Source: CAD feature listing. Evaluate the final solid. Frame: model axes, mm. A direction names the side the tool comes from. Give positions to 0.01 mm unless a question says otherwise; leave off trailing zeros. Loops run counter-clockwise (first coordinate to the right, second up) from the corner with the lowest first, then second, coordinate; pieces in that order, holes last.
from build123d import *

# Parameters (mm, degrees)
SKETCH_1_W          = 110
SKETCH_1_H          = 110
EXTRUDE_1_DEPTH     = 9
SKETCH_2_R          = 6.2
CUT_EXTRUDE_1_DEPTH = 9
SKETCH_10_W         = 8
SKETCH_10_H         = 8
CUT_EXTRUDE_3_DEPTH = 10
SKETCH_9_W          = 110
SKETCH_9_H          = 15
CUT_EXTRUDE_4_DEPTH = 10
FILLET_1_R          = 10
SKETCH_11_W         = 8
SKETCH_11_H         = 3
CUT_EXTRUDE_5_DEPTH = 10
SKETCH_12_R         = 1.7
CUT_EXTRUDE_6_DEPTH = 10


with BuildPart() as part:
    # 草图1 → 凸台-拉伸1 (new body)
    with BuildSketch(Plane(origin=(0, 0, 0), x_dir=(1, 0, 0), z_dir=(0, 1, 0))):
        with BuildLine():
            Line((-98.584118364, 105), (98.584118364, 105))
            ThreePointArc((98.584118364, 105), (103.984134744, 103.416639656), (107.674116766, 99.167964619))
            Line((107.674116766, 99.167964619), (147.029996803, 13.335929237))
            ThreePointArc((147.029996803, 13.335929237), (148.644315385, 2.139042389), (143.925625878, -8.142507538))
            Line((143.925625878, -8.142507538), (92.989084735, -66.571253769))
            ThreePointArc((92.989084735, -66.571253769), (89.591770698, -69.102541889), (85.451271796, -70))
            Line((85.451271796, -70), (50, -70))
            Line((50, -70), (-55, -70))
            Line((-55, -70), (-85.451271796, -70))
            ThreePointArc((-85.451271796, -70), (-89.591770698, -69.102541889), (-92.989084735, -66.571253769))
            Line((-92.989084735, -66.571253769), (-143.925625878, -8.142507538))
            ThreePointArc((-143.925625878, -8.142507538), (-148.644315385, 2.139042389), (-147.029996803, 13.335929237))
            Line((-147.029996803, 13.335929237), (-107.674116766, 99.167964619))
            ThreePointArc((-107.674116766, 99.167964619), (-103.984134744, 103.416639656), (-98.584118364, 105))
        make_face()
        Rectangle(SKETCH_1_W, SKETCH_1_H, mode=Mode.SUBTRACT)
    extrude(amount=EXTRUDE_1_DEPTH)

    # 草图2 → 切除-拉伸1 (cut)
    with BuildSketch(Plane(origin=(0, 9, 0), x_dir=(1, 0, 0), z_dir=(0, 1, 0))):
        with Locations(Location((-128.85, 5, 0), (0, 0, 270))):
            Circle(SKETCH_2_R)
        with Locations(Location((128.85, 5, 0), (0, 0, 270))):
            Circle(SKETCH_2_R)
    extrude(amount=-CUT_EXTRUDE_1_DEPTH, mode=Mode.SUBTRACT)

    # 草图10 → 切除-拉伸3 (cut)
    with BuildSketch(Plane(origin=(0, 9, 0), x_dir=(1, 0, 0), z_dir=(0, 1, 0))):
        with Locations((-59, 0)):
            Rectangle(SKETCH_10_W, SKETCH_10_H)
        with Locations((0, 59)):
            Rectangle(SKETCH_10_W, SKETCH_10_H)
        with Locations((59, 0)):
            Rectangle(SKETCH_10_W, SKETCH_10_H)
        with Locations((0, -59)):
            Rectangle(SKETCH_10_W, SKETCH_10_H)
    extrude(amount=-CUT_EXTRUDE_3_DEPTH, mode=Mode.SUBTRACT)

    # 草图9 → 切除-拉伸4 (cut)
    with BuildSketch(Plane.XZ):
        with Locations((0, 62.5)):
            Rectangle(SKETCH_9_W, SKETCH_9_H)
    extrude(amount=-CUT_EXTRUDE_4_DEPTH, mode=Mode.SUBTRACT)

    # 圆角1
    fillet_1_edges = [part.edges().sort_by_distance(p)[0] for p in [
        (55, 4.5, 70),
        (-55, 4.5, 70),
    ]]
    fillet(fillet_1_edges, radius=FILLET_1_R)

    # 草图11 → 切除-拉伸5 (cut)
    with BuildSketch(Plane(origin=(0, 9, 0), x_dir=(1, 0, 0), z_dir=(0, 1, 0))):
        with Locations((71, 4.5)):
            Rectangle(SKETCH_11_W, SKETCH_11_H)
        with Locations((71, -4.5)):
            Rectangle(SKETCH_11_W, SKETCH_11_H)
        with Locations((-71, 4.5)):
            Rectangle(SKETCH_11_W, SKETCH_11_H)
        with Locations((-71, -4.5)):
            Rectangle(SKETCH_11_W, SKETCH_11_H)
    extrude(amount=-CUT_EXTRUDE_5_DEPTH, mode=Mode.SUBTRACT)

    # 草图12 → 切除-拉伸6 (cut)
    with BuildSketch(Plane(origin=(0, 9, 0), x_dir=(1, 0, 0), z_dir=(0, 1, 0))):
        with Locations(Location((-128.85, 15.5, 0), (0, 0, 270))):
            Circle(SKETCH_12_R)
        with Locations(Location((-118.35, 5, 0), (0, 0, 270))):
            Circle(SKETCH_12_R)
        with Locations(Location((-128.85, -5.5, 0), (0, 0, 270))):
            Circle(SKETCH_12_R)
        with Locations(Location((-139.35, 5, 0), (0, 0, 270))):
            Circle(SKETCH_12_R)
        with Locations(Location((139.35, 5, 0), (0, 0, 270))):
            Circle(SKETCH_12_R)
        with Locations(Location((128.85, -5.5, 0), (0, 0, 270))):
            Circle(SKETCH_12_R)
        with Locations(Location((118.35, 5, 0), (0, 0, 270))):
            Circle(SKETCH_12_R)
        with Locations(Location((128.85, 15.5, 0), (0, 0, 270))):
            Circle(SKETCH_12_R)
    extrude(amount=-CUT_EXTRUDE_6_DEPTH, mode=Mode.SUBTRACT)


solid = part.part
1) Contact query for flat-ended pins moving along their axis: P1, Ø2.5, axis at y = 6, z = -4, coming from the -X side; P2, Ø2.5, axis at x = -59.5, y = 4.5, coming from the +Z side; P3, Ø5, axis at y = 7, z = 4, coming from the +X side; P4, Ø0.9, axis at y = 4.5, z = 5, coming from the +X side. Output: stop coordinate, or through.
Checks:
P1: stops at x = -148.85
P2: stops at z = 69.05
P3: stops at x = 147.76
P4: stops at x = 146.42
2) Cut plane D-D (z = 24). Return loops of the section in (x, y).
Checks:
outline: (-130.1, 0) - (-55, 0) - (-55, 9) - (-130.1, 9) - close; (55, 0) - (130.1, 0) - (130.1, 9) - (55, 9) - close
3) Pull-direction query (X, two-part tool) for faces 1 (the flat face through (-31, 0, -58)), 2 (the flat face through (-59, 5, 4)), 3 (the flat face through (71, 5, 3)), 4 (the cylindrical face through (-89.537, 4.437, 69.127)); classes: released by +X, released by -X, zero draft, split by the parting line, or undercut.
Checks:
face 1: zero draft
face 2: undercut
face 3: undercut
face 4: released by -X
4) Cut plane C-C (x = 39). Return loops of the section in (y, z).
Checks:
outline: (0, -105) - (9, -105) - (9, -55) - (0, -55) - close
5) Reachability of faces 5 (the flat face through (-118.101, 4.437, 37.766)), 6 (the flat face through (55, 4, -29)), 7 (the flat face through (59, 5, -4)) from +Z, -Z, +X, -X, +Y, -Y: full face, straight path, thin tool, end or side. Return the list, or none.
Checks:
face 5: +Z, -X, +Y, -Y
face 6: +Z, +Y, -Y
face 7: +Y, -Y
6) Cut plane B-B (y = 5). State how many separate pieces and enclosed holes the cut face has, and give its area (3 significant figures).
Checks:
separate pieces: 1
enclosed holes: 14
area: 29,500 mm2
7) Cut plane A-A (z = -34). Return loops of the section in (x, y).
Checks:
outline: (-137.56, 0) - (-55, 0) - (-55, 9) - (-137.56, 9) - close; (55, 0) - (137.56, 0) - (137.56, 9) - (55, 9) - close
8) Ray query, probe 1 along X at (y, z) = (5.5, -26.5); probe 2 along Z at (x, y) = (-74, 5); probe 3 along X at (y, z) = (5, 5.5). Return the intervals inside material, ascending.
Checks:
probe 1: x = -140.99 to -55, 55 to 140.99
probe 2: z = -105 to -6, -3 to 3, 6 to 70
probe 3: x = -145.87 to -130.55, -127.15 to -75, -67 to -55, 55 to 67, 75 to 127.15, 130.55 to 145.87
